The model under review builds one solid part; all positions refer to its coordinate system, in mm. A direction names the side the tool comes from. Coordinates: 2 decimals unless noted, no trailing zeros. Order: outer loops, then holes, each group sorted by start corner. A loop starts at its lowest first (then second) coordinate and runs counter-clockwise, first axis right, second up. Notation, with made-up numbers: M 44,22.25 L 59,22.25 A9 ccw 59,33.25 Z; hole C 63,67 d3. An arc over 180 degrees is marked long. Answer in a Markdown table with one row per item.
from build123d import *

# Parameters (mm, degrees)
SKETCH1_W                     = 120
SKETCH1_H                     = 100
BOSS_EXTRUDE1_DEPTH           = 10
SKETCH2_W                     = 13
SKETCH2_H                     = 15
CUT_EXTRUDE1_DEPTH            = 35
SKETCH3_W                     = 7.5
SKETCH3_H                     = 7.5
SKETCH3_W_2                   = 14
CUT_EXTRUDE2_DEPTH            = 7.5
SKETCH4_R                     = 1.5
CUT_EXTRUDE3_DEPTH            = 75.5
CBORE_FOR_M3_SHCS_D           = 3.4
CBORE_FOR_M3_SHCS_DEPTH       = 23
CBORE_FOR_M3_SHCS_CBORE_D     = 6.5
CBORE_FOR_M3_SHCS_CBORE_DEPTH = 3
CBORE_FOR_M3_SHCS_TIP         = 1.021463052


with BuildPart() as part:
    # Sketch1 → Boss-Extrude1 (new body)
    with BuildSketch(Plane(origin=(0, 0, 0), x_dir=(1, 0, 0), z_dir=(0, 1, 0))):
        Rectangle(SKETCH1_W, SKETCH1_H)
    extrude(amount=BOSS_EXTRUDE1_DEPTH)

    # Sketch2 → Cut-Extrude1 (cut)
    with BuildSketch(Plane.XY.offset(50)):
        with Locations((-36, 0)):
            Rectangle(SKETCH2_W, SKETCH2_H)
        with Locations((-12, 0)):
            Rectangle(SKETCH2_W, SKETCH2_H)
        with Locations((12, 0)):
            Rectangle(SKETCH2_W, SKETCH2_H)
        with Locations((36, 0)):
            Rectangle(SKETCH2_W, SKETCH2_H)
    extrude(amount=-CUT_EXTRUDE1_DEPTH, mode=Mode.SUBTRACT)

    # Sketch3 → Cut-Extrude2 (cut)
    with BuildSketch(Plane.XY.offset(50)):
        with Locations((-22.25, 3.75)):
            Rectangle(SKETCH3_W, SKETCH3_H)
        with Locations((1.75, 3.75)):
            Rectangle(SKETCH3_W, SKETCH3_H)
        with Locations((25.75, 3.75)):
            Rectangle(SKETCH3_W, SKETCH3_H)
        with Locations((53, 3.75)):
            Rectangle(SKETCH3_W_2, SKETCH3_H)
    extrude(amount=-CUT_EXTRUDE2_DEPTH, mode=Mode.SUBTRACT)

    # Sketch4 → Cut-Extrude3 (cut)
    with BuildSketch(Plane(origin=(46, 0, 0), x_dir=(0, 0, -1), z_dir=(1, 0, 0))):
        with Locations((-46.25, 3.75)):
            Circle(SKETCH4_R)
    extrude(amount=-CUT_EXTRUDE3_DEPTH, mode=Mode.SUBTRACT)

    # CBORE for M3 SHCS
    with Locations(Plane(origin=(-676.293536786, 10, -1323.282701689), x_dir=(1, 0, 0), z_dir=(0, 1, 0))):
        with Locations((731.293536786, -1281.282701689), (731.293536786, -1359.282701689), (621.293536786, -1281.282701689), (621.293536786, -1365.282701689), (621.293536786, -1323.282701689), (731.293536786, -1320.282701689)):
            CounterBoreHole(CBORE_FOR_M3_SHCS_D / 2, CBORE_FOR_M3_SHCS_CBORE_D / 2, CBORE_FOR_M3_SHCS_CBORE_DEPTH, depth=CBORE_FOR_M3_SHCS_DEPTH)
            with Locations((0, 0, -(CBORE_FOR_M3_SHCS_DEPTH + CBORE_FOR_M3_SHCS_TIP / 2))):  # 118° drill point
                Cone(0, CBORE_FOR_M3_SHCS_D / 2, CBORE_FOR_M3_SHCS_TIP, mode=Mode.SUBTRACT)


solid = part.part
(1) The part is to be moulded in two halves that separate along Z. For faces 4 (the cylindrical face through (44.27, 3.82, 47.75)), 5 (the flat face through (12, 4, 15)), 6 (the flat face through (-1, 0, -12)), say which applies: +Z half, -Z half, draft (parallel to the pull), parting line (faces both ways), or undercut.
Report:
| item | result |
|---|---|
| face 4 | undercut |
| face 5 | +Z half |
| face 6 | draft |
(2) Take a section at A-A (z = -42). Write out the cut boundary in (x, y), then the cut area to 3 significant figures.
Report:
| item | result |
|---|---|
| outline | M -60,0 L -56.7,0 L -56.7,7 L -58.25,7 L -58.25,10 L -60,10 Z; M -53.3,0 L 53.3,0 L 53.3,7 L 51.75,7 L 51.75,10 L -51.75,10 L -51.75,7 L -53.3,7 Z; M 56.7,0 L 60,0 L 60,10 L 58.25,10 L 58.25,7 L 56.7,7 Z |
| area | 1,110 mm^2 |
(3) Insertion check: P1, Ø6, axis at x = -43.5, z = 29, coming from the -Y side; P2, Ø5, axis at y = 3.75, z = 46.25, coming from the +X side; P3, Ø2, axis at x = 56, z = 35.5, coming from the +Y side; P4, Ø2.5, axis at y = 3.75, z = 46.25, coming from the +X side. Each pin has a flat end and moves straight along its axis. Give the tip position at first contact, or say it passes through.
Report:
| item | result |
|---|---|
| P1 | y = 0 |
| P2 | x = 46 |
| P3 | y = 7 |
| P4 | x = -42.5 |
(4) To check wall thickness, follow line 1 (Z direction, x = -55, y = 9.2); line 2 (X direction, y = 4.5, z = -42); line 3 (Y direction, x = 20.9, z = 46.25). State the ranges of each line that lie inside material, in increasing order. Write a range as [from, to].
Report:
| item | result |
|---|---|
| line 1 | [-50, -45.25], [-38.75, -3.25], [3.25, 38.75], [45.25, 50] |
| line 2 | [-60, -56.7], [-53.3, 53.3], [56.7, 60] |
| line 3 | [0, 2.25], [5.25, 10] |
(5) Take a section at C-C (z = 36). Write out the cut boundary in (x, y).
Report:
| item | result |
|---|---|
| outline | M -60,0 L -42.5,0 L -42.5,7.5 L -29.5,7.5 L -29.5,0 L -18.5,0 L -18.5,7.5 L -5.5,7.5 L -5.5,0 L 5.5,0 L 5.5,7.5 L 18.5,7.5 L 18.5,0 L 29.5,0 L 29.5,7.5 L 42.5,7.5 L 42.5,0 L 53.3,0 L 53.3,7 L 51.75,7 L 51.75,10 L -60,10 Z; M 56.7,0 L 60,0 L 60,10 L 58.25,10 L 58.25,7 L 56.7,7 Z |
(6) Take a section at B-B (x = 55). State how many separate pieces and enclosed holes the cut face has, then the cut area to 3 significant figures.
Report:
| item | result |
|---|---|
| separate pieces | 4 |
| enclosed holes | 0 |
| area | 814 mm^2 |
(7) Machinability: for faces 1 (the flat face through (-1, 5, -50)), 2 (the cylindrical face through (51.753, 8.521, -3.143)), 3 (the flat face through (-22, 4, 42.5)), which of the approach directions +Z, -Z, +X, -X, +Y, -Y give a long, thin tool a straight path to every point of the face, cutting with its end or side? Answer none if there is none.
Report:
| item | result |
|---|---|
| face 1 | -Z, +X, -X, +Y, -Y |
| face 2 | +Y |
| face 3 | +Z, -Y |
